Part model, mm, in its own coordinate system. Face numbers are marked on the shaded views. A direction names the side the tool comes from. Coordinates: 2 decimals unless noted, no trailing zeros. Loops run counter-clockwise (first coordinate to the right, second up) from the corner with the lowest first, then second, coordinate; pieces in that order, holes last. Notation, with made-up numbers: (62, 73.5) -> (72, 73.5) arc R14 cw to (72, 85.5) -> close; hole circle Ø5 at (2.25, 77). An arc over 180 degrees is marked (long way). One line per question, with ' | ' between items. Start each with the question number.
1) Two-plate mould, pull along X, no slides. Class the marked faces 3, 4 and 5: released by +X, released by -X, zero draft, split by the parting line, or undercut.
2) 3-axis set-ups, long thin cutter, end or side, ignore diameter. For the marked faces 1 and 2: which of +Z, -Z, +X, -X, +Y, -Y reach the whole face in a straight line?
3) Cut at B-B (y = 1.25). List the corners of the cut face in (x, z).
4) Probe L1, parallel to X at y = 2.75, z = 10.5; L2, parallel to Z at x = -3.25, y = 7.5; L3, parallel to Z at x = -2, y = 3. List the from-to ranges inside material, lowest first. Write a range as from..to.
5) Cut at A-A (z = 2.25). List the corners of the cut face in (x, y), plus the area to 3 significant figures.
6) Cut at D-D (z = -4.75). List the corners of the cut face in (x, y).
7) Cut at C-C (x = 0). List the corners of the cut face in (y, z).
8) Drop flat-ended pins along their axis: pin 1 (2 mm diameter, centred on x = -3.5, z = -0.5, fed in from +Y); pin 2 (10 mm diameter, centred on x = 3.5, z = 0.5, fed in from +Y). Give the stop position or say it passes through.
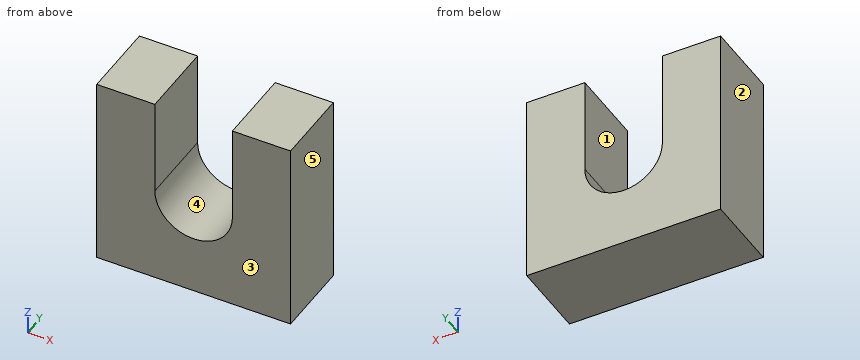
from build123d import *

# Parameters (mm, degrees)
BOSS_EXTRUDE1_DEPTH = 10.16


with BuildPart() as part:
    # Sketch1 → Boss-Extrude1 (new body)
    with BuildSketch(Plane(origin=(0, 0, 0), x_dir=(1, 0, 0), z_dir=(0, 1, 0))):
        with BuildLine():
            Line((-5.08, -12.7), (-5.08, 0))
            ThreePointArc((-5.08, 0), (0, 5.08), (5.08, 0))
            Line((5.08, 0), (5.08, -12.7))
            Line((5.08, -12.7), (12.7, -12.7))
            Line((12.7, -12.7), (12.7, 12.7))
            Line((12.7, 12.7), (-12.7, 12.7))
            Line((-12.7, 12.7), (-12.7, -12.7))
            Line((-12.7, -12.7), (-5.08, -12.7))
        make_face()
    extrude(amount=BOSS_EXTRUDE1_DEPTH)


solid = part.part
Reported:
1) face 3: zero draft | face 4: undercut | face 5: released by +X
2) face 1: +Z, +Y, -Y | face 2: +Z, -Z, -X, +Y, -Y
3) outline: (-12.7, -12.7) -> (12.7, -12.7) -> (12.7, 12.7) -> (5.08, 12.7) -> (5.08, 0) arc R5.08 cw to (-5.08, 0) -> (-5.08, 12.7) -> (-12.7, 12.7) -> close
4) L1: x = -12.7..-5.08, 5.08..12.7 | L2: z = -12.7..-3.9 | L3: z = -12.7..-4.67
5) outline: (-12.7, 0) -> (-5.08, 0) -> (-5.08, 10.16) -> (-12.7, 10.16) -> close; (5.08, 0) -> (12.7, 0) -> (12.7, 10.16) -> (5.08, 10.16) -> close | area: 155 mm²
6) outline: (-12.7, 0) -> (-1.8, 0) -> (-1.8, 10.16) -> (-12.7, 10.16) -> close; (1.8, 0) -> (12.7, 0) -> (12.7, 10.16) -> (1.8, 10.16) -> close
7) outline: (0, -12.7) -> (10.16, -12.7) -> (10.16, -5.08) -> (0, -5.08) -> close
8) pin 1: passes through | pin 2: stops at y = 10.16
